Autodesk Inventor part; units mm, degrees
ref_plane "ANBAU_XY" through (0, 0, -4) normal (0, 0, 1) x (1, 0, 0)
ref_plane "ANBAU_YZ" through (0, 0, -4) normal (1, 0, 0) x (0, 1, 0)
ref_plane "ANBAU_ZX" through (0, 0, -4) normal (0, 1, 0) x (0, 0, 1)
sketch "Sketch_1" plane through (0, 0, 0) normal (1, 0, 0) x (0, 1, 0)
  line L0 (0, -4) -> (0, 0)
  line L1 (12.5, 0) -> (12.5, -4)
  line L2 (12.5, -4) -> (17.5, -4)
  line L3 (17.5, -4) -> (17.5, 0)
  line L4 (17.5, 0) -> (16.4679, 0)
  line L5 (16.4679, 0) -> (16.2, -1)
  line L6 (16.2, -1) -> (13.5, -1)
  line L7 (13.5, -1) -> (12.5, 0)
revolve "Revolution1" add sketch "Sketch_1" angle 360 about axis through (0, 0, -4) along (0, 0, -1)
ref_plane "ANBAU_XY" through (0, 0, -4) normal (0, 0, 1) x (1, 0, 0)
ref_plane "ANBAU_YZ" through (0, 0, -4) normal (1, 0, 0) x (0, 1, 0)
ref_plane "ANBAU_ZX" through (0, 0, -4) normal (0, 1, 0) x (0, 0, 1)
properties part number "247465 FEN-80-SD---(SD)"
Can you work these out from the model? Positions are in its coordinate system, mm. Coordinates: 2 decimals unless noted, no trailing zeros. Loops run counter-clockwise (first coordinate to the right, second up) from the corner with the lowest first, then second, coordinate; pieces in that order, holes last. Notation, with made-up numbers: (-35.75, 38.25) -> (5.25, 38.25) arc R29 cw to (5.25, 62.25) -> close; hole circle Ø11 at (-19, 58). An arc over 180 degrees is marked (long way). Answer as a JSON object with one key per item and string values.
1) For P1, Ø1, axis at x = -12, z = -2, coming from the -Y side; P2, Ø1, axis at x = 12, z = -1, coming from the +Y side, each with a flat end and sliding along its axis, tell me the tip position at first contact or that it passes through.
Results:
{"P1": "stops at y = -13.19", "P2": "stops at y = 13.19"}
2) Thinking about a two-plate mould opening in Y: for faces 1 (the face through (-12, -12, 0)), 2 (the face through (10.648, -13.887, -1.972)), 3 (the face through (13.3, -3.7, -1)), 4 (the face through (3.755, 11.923, -2.028)), which applies, pulls with the +Y half, pulls with the -Y half, needs draft (parallel to the pull), parting line crosses it, or undercut?
Results:
{"face 1": "needs draft", "face 2": "parting line crosses it", "face 3": "undercut", "face 4": "undercut"}
3) Imagine slicing it at A-A (y = 0). Please give me the cut outline in (x, z).
Results:
{"outline": "(-17.5, -4) -> (-12.5, -4) -> (-12.5, 0) -> (-13.5, -1) -> (-16.2, -1) -> (-16.47, 0) -> (-17.5, 0) -> close; (12.5, -4) -> (17.5, -4) -> (17.5, 0) -> (16.47, 0) -> (16.2, -1) -> (13.5, -1) -> (12.5, 0) -> close"}
4) Imagine slicing it at C-C (z = -0.6). Please give me the cut outline in (x, y).
Results:
{"outline": "circle Ø35 at (0, 0); circle Ø26.2 at (0, 0); hole circle Ø32.61 at (0, 0); hole circle Ø25 at (0, 0)"}
5) If I drill on line 1 (X direction, y = 4, z = -0.3); line 2 (X direction, y = 0, z = -1.4); line 3 (Y direction, x = 9.5, z = -0.4), over which ranges is the centre line in solid material (lowest first)?
Results:
{"line 1": "x = -17.04 to -15.89, -12.16 to -11.84, 11.84 to 12.16, 15.89 to 17.04", "line 2": "x = -17.5 to -12.5, 12.5 to 17.5", "line 3": "y = -14.7 to -13.32, -8.73 to -8.12, 8.12 to 8.73, 13.32 to 14.7"}
